Design review of the part built by this model. Coordinates are the model's own, in mm. Face numbers are marked on the shaded views. A direction names the side the tool comes from. Give positions to 0.01 mm unless a question says otherwise; leave off trailing zeros. Write each loop counter-clockwise with the first axis right and the second up, starting at its lowest first coordinate (ties: lowest second). Pieces come first, ordered by that corner, then holes. Notation, with made-up numbers: (85.25, 8.5) -> (107.25, 8.5) arc R16 ccw to (107.25, 13.5) -> close; hole circle Ø9 at (86, 88). An arc over 180 degrees is marked (long way). Write each question's results on one line, items separated by ' | '. Start each with the question number.
(1) To check wall thickness, follow probe 1 along X at (y, z) = (-8, 0); probe 2 along Y at (x, z) = (3.75, 0); probe 3 along Y at (x, z) = (12, -0.5). State the ranges of each line that lie inside material, in increasing order.
(2) Take a section at D-D (y = -11.25). State the section outline as (x, z) points, plus the area to 3 significant figures.
(3) Take a section at B-B (z = 0). State the section outline as (x, y) points, plus the area to 3 significant figures.
(4) For the marked faces 4, 5, 6 and 7, list the 3-axis set-ups (+Z, -Z, +X, -X, +Y, -Y) from which the entire face can be reached by the end or side of a thin tool; tool diameter is ignored.
(5) Take a section at A-A (y = 0). State the section outline as (x, z) points.
(6) Clearance check with flat-ended pins moving along their axes: pin 1 (9.5 mm diameter, centred on y = 4.5, z = 2, fed in from +X); pin 2 (1.5 mm diameter, centred on x = 13, y = 8, fed in from -Z); pin 3 (4 mm diameter, centred on x = 32.5, y = -8, fed in from +Z). State where each tip first meets the part, or that it passes through.
(7) Take a section at C-C (x = 6). State the section outline as (y, z) points, plus the area to 3 significant figures.
(8) Mouldability with a two-part tool opening along X and no side actions: class the marked faces 1, 2 and 3 as released by +X, released by -X, zero draft, split by the parting line, or undercut.
from build123d import *

# Parameters (mm, degrees)
CROQUIS1_R                 = 14.5
SALIENTE_EXTRUIR1_DEPTH    = 46
CROQUIS2_R                 = 4
CORTAR_EXTRUIR1_DEPTH      = 8
CROQUIS3_R                 = 11
CORTAR_EXTRUIR2_DEPTH      = 15.5
CORTAR_EXTRUIR2_DEPTH_BACK = 15.5
CROQUIS4_W                 = 19
CROQUIS4_H                 = 19
CORTAR_EXTRUIR3_DEPTH      = 10
CROQUIS5_W                 = 19
CROQUIS5_H                 = 2.5
SALIENTE_EXTRUIR2_DEPTH    = 28
CROQUIS7_R                 = 11.15
SALIENTE_EXTRUIR3_DEPTH    = 2.5


with BuildPart() as part:
    # Croquis1 → Saliente-Extruir1 (new body)
    with BuildSketch(Plane(origin=(0, 0, 0), x_dir=(0, 0, -1), z_dir=(1, 0, 0))):
        Circle(CROQUIS1_R)
    extrude(amount=SALIENTE_EXTRUIR1_DEPTH)

    # Croquis2 → Cortar-Extruir1 (cut)
    with BuildSketch(Plane.ZY):
        Circle(CROQUIS2_R)
    extrude(amount=-CORTAR_EXTRUIR1_DEPTH, mode=Mode.SUBTRACT)

    # Croquis3 → Cortar-Extruir2 (cut, two sides)
    with BuildSketch(Plane(origin=(0, 0, 0), x_dir=(1, 0, 0), z_dir=(0, 1, 0))) as cortar_extruir2_sk:
        with Locations((21, 0)):
            Circle(CROQUIS3_R)
    extrude(amount=CORTAR_EXTRUIR2_DEPTH, mode=Mode.SUBTRACT)
    extrude(cortar_extruir2_sk.sketch, amount=-CORTAR_EXTRUIR2_DEPTH_BACK, mode=Mode.SUBTRACT)

    # Croquis4 → Cortar-Extruir3 (cut)
    with BuildSketch(Plane(origin=(46, 0, 0), x_dir=(0, 0, -1), z_dir=(1, 0, 0))):
        Rectangle(CROQUIS4_W, CROQUIS4_H)
    extrude(amount=-CORTAR_EXTRUIR3_DEPTH, mode=Mode.SUBTRACT)

    # Croquis5 → Saliente-Extruir2 (add)
    with BuildSketch(Plane(origin=(36, 0, 0), x_dir=(0, 0, -1), z_dir=(1, 0, 0))):
        Rectangle(CROQUIS5_W, CROQUIS5_H)
    extrude(amount=-SALIENTE_EXTRUIR2_DEPTH)

    # Croquis7 → Saliente-Extruir3 (add)
    with BuildSketch(Plane.XZ.offset(1.25)):
        with Locations((21, 0)):
            Circle(CROQUIS7_R)
    extrude(amount=-SALIENTE_EXTRUIR3_DEPTH)


solid = part.part
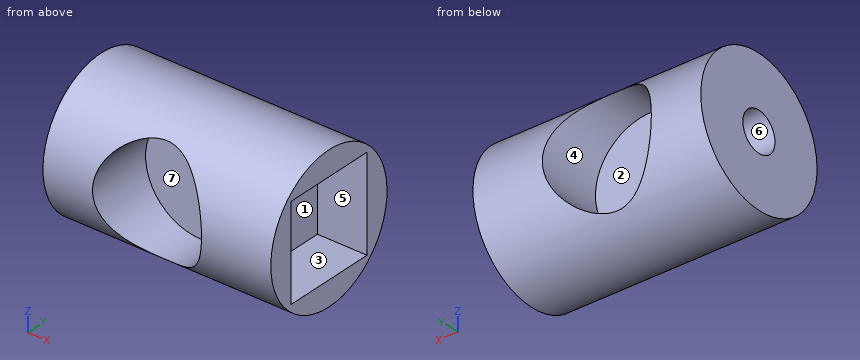
Report:
1) probe 1: 0 to 10, 32 to 36 | probe 2: -14.5 to -4, 4 to 14.5 | probe 3: -1.25 to 1.25
2) outline: (0, -9.15) -> (14.89, -9.15) arc R11 cw to (14.89, 9.15) -> (0, 9.15) -> close; (27.11, -9.15) -> (46, -9.15) -> (46, 9.15) -> (27.11, 9.15) arc R11 cw to start | area: 492 mm2
3) outline: (0, -14.5) -> (10, -14.5) -> (10, -1.25) -> (32, -1.25) -> (32, -14.5) -> (46, -14.5) -> (46, -9.5) -> (36, -9.5) -> (36, 9.5) -> (46, 9.5) -> (46, 14.5) -> (32, 14.5) -> (32, 1.25) -> (10, 1.25) -> (10, 14.5) -> (0, 14.5) -> (0, 4) -> (8, 4) -> (8, -4) -> (0, -4) -> close | area: 497 mm2
4) face 4: +Y | face 5: +X | face 6: -X | face 7: -Y
5) outline: (0, -14.5) -> (46, -14.5) -> (46, -9.5) -> (36, -9.5) -> (36, 9.5) -> (46, 9.5) -> (46, 14.5) -> (0, 14.5) -> (0, 4) -> (8, 4) -> (8, -4) -> (0, -4) -> close
6) pin 1: x = 36 | pin 2: z = -12.56 | pin 3: z = 13.2
7) outline: circle Ø29 at (0, 0); hole circle Ø8 at (0, 0) | area: 610 mm2
8) face 1: released by +X | face 2: undercut | face 3: zero draft
